from build123d import *

# Parameters (mm, degrees)
SKETCH1_R           = 13.499973
BOSS_EXTRUDE1_DEPTH = 23.0000048
SKETCH2_R           = 2.5
BOSS_EXTRUDE2_DEPTH = 10
SKETCH3_R           = 1.499997
BOSS_EXTRUDE3_DEPTH = 2
SKETCH4_R           = 1.524
SKETCH4_R_2         = 1.5
CUT_EXTRUDE1_DEPTH  = 2


with BuildPart() as part:
    # Sketch1 → Boss-Extrude1 (new body)
    with BuildSketch(Plane(origin=(0, 0, 0), x_dir=(1, 0, 0), z_dir=(0, 1, 0))):
        with Locations(Location((0, 0, 0), (0, 0, 270))):
            Circle(SKETCH1_R)
    extrude(amount=BOSS_EXTRUDE1_DEPTH)

    # Sketch2 → Boss-Extrude2 (add)
    with BuildSketch(Plane(origin=(0, 23.0000048, 0), x_dir=(1, 0, 0), z_dir=(0, 1, 0))):
        with Locations(Location((0, 0, 0), (0, 0, 270))):
            Circle(SKETCH2_R)
    extrude(amount=BOSS_EXTRUDE2_DEPTH)

    # Sketch3 → Boss-Extrude3 (add)
    with BuildSketch(Plane.XZ):
        with Locations(Location((0, 0, 0), (0, 0, 90))):
            Circle(SKETCH3_R)
    extrude(amount=BOSS_EXTRUDE3_DEPTH)

    # Sketch4 → Cut-Extrude1 (cut)
    with BuildSketch(Plane.XZ):
        with Locations((0, 12.5000004)):
            Circle(SKETCH4_R)
        with Locations(Location((9.4999937, 0, 0), (0, 0, 270))):
            Circle(SKETCH4_R_2)
        with Locations(Location((-9.4999937, 0, 0), (0, 0, 90))):
            Circle(SKETCH4_R_2)
        with Locations((0, -12.5000004)):
            Circle(SKETCH4_R)
    extrude(amount=-CUT_EXTRUDE1_DEPTH, mode=Mode.SUBTRACT)


solid = part.part
The model under review builds one solid part; all positions refer to its coordinate system, in mm. A direction names the side the tool comes from. Give positions to 0.01 mm unless a question says otherwise; leave off trailing zeros. Loops run counter-clockwise (first coordinate to the right, second up) from the corner with the lowest first, then second, coordinate; pieces in that order, holes last. Notation, with made-up numbers: (40.5, -8.5) -> (96.5, -8.5) arc R7 cw to (96.5, -1.5) -> close; hole circle Ø10 at (63, -0.75). An arc over 180 degrees is marked (long way). Put each result on its own line as item: value. Start each with the question number.
1. Clearance check with flat-ended pins moving along their axes: P1, Ø2.5, axis at x = -9.5, z = 0, coming from the -Y side; P2, Ø3, axis at y = 28, z = -2.5, coming from the +X side; P3, Ø4, axis at y = 23, z = 2.5, coming from the -X side. State where each tip first meets the part, or that it passes through.
2. We need section C-C on y = 8.5. State the section outline as (x, z) points.
3. Mouldability with a two-part tool opening along Z and no side actions: class faces 4 (the face through (0.048, 0.986, -10.977)), 5 (the face through (4.055, 11.339, 12.877)), 6 (the face through (0, 0, 3)), 7 (the face through (10, 2, 0)) as released by +Z, released by -Z, zero draft, split by the parting line, or undercut.
4. We need section D-D on y = 26. State the section outline as (x, z) points, then the cut area to 3 significant figures.
5. Wall thickness on probe 1 along X at (y, z) = (1.4, 0); probe 2 along Y at (x, z) = (7.25, -1); probe 3 along X at (y, z) = (12.5, 10.75): over which ranges is each line inside the solid? List them lowest first.
6. We need section B-B on x = 0. State the section outline as (y, z) points, then the cut area to 3 significant figures.
7. For faces 1 (the face through (10.765, 0.986, -0.806)), 2 (the face through (0, 33, 0)), 3 (the face through (-2.44, 27.93, -0.54)), list the 3-axis set-ups (+Z, -Z, +X, -X, +Y, -Y) from which the entire face can be reached by the end or side of a thin tool; tool diameter is ignored.
8. We need section A-A on z = 0. State the section outline as (x, y) points.
Determined:
1. P1: y = 2
1. P2: x = 2.29
1. P3: x = -13.49
2. outline: circle Ø27 at (0, 0)
3. face 4: undercut
3. face 5: split by the parting line
3. face 6: zero draft
3. face 7: undercut
4. outline: circle Ø5 at (0, 0)
4. area: 19.6 mm^2
5. probe 1: -13.5 to -11, -8 to 8, 11 to 13.5
5. probe 2: 0 to 23
5. probe 3: -8.17 to 8.17
6. outline: (-2, -1.5) -> (0, -1.5) -> (0, -10.98) -> (2, -10.98) -> (2, -13.5) -> (23, -13.5) -> (23, -2.5) -> (33, -2.5) -> (33, 2.5) -> (23, 2.5) -> (23, 13.5) -> (2, 13.5) -> (2, 10.98) -> (0, 10.98) -> (0, 1.5) -> (-2, 1.5) -> close
6. area: 667 mm^2
7. face 1: -Y
7. face 2: +Z, -Z, +X, -X, +Y
7. face 3: +Y
8. outline: (-13.5, 0) -> (-11, 0) -> (-11, 2) -> (-8, 2) -> (-8, 0) -> (-1.5, 0) -> (-1.5, -2) -> (1.5, -2) -> (1.5, 0) -> (8, 0) -> (8, 2) -> (11, 2) -> (11, 0) -> (13.5, 0) -> (13.5, 23) -> (2.5, 23) -> (2.5, 33) -> (-2.5, 33) -> (-2.5, 23) -> (-13.5, 23) -> close
